Geometry: see drawing. Coordinates: mm, zero at the bounding-box minimum. A direction names the side the tool comes from. Coordinates: 2 decimals unless noted, no trailing zeros. Write each loop counter-clockwise with the first axis right and the second up, starting at its lowest first coordinate (ties: lowest second). Pieces come first, ordered by that corner, then holes. Notation, with made-up numbers: (58.25, 49.25) - (108.25, 49.25) arc R5 ccw to (108.25, 57.25) - close; hole circle Ø5 at (48.5, 77.5). An arc over 180 degrees is marked (long way). One line per question, with ' | ' between items. Start each with the question number.
Q1. Line query: line 1 (Z direction, x = 5.25, y = 0.85) (1 decimal); line 2 (X direction, y = 1.55, z = 7.25) (1 decimal); line 3 (X direction, y = 1, z = 3.25) (1 decimal). Output: solid intervals per line, ascending.
Q2. Cut plane A-A, the plane y = 0.55. Return loops of the section in (x, z) (1 decimal).
Q3. Draft query along X for the marked faces 1, 2, 3 and 4. Return one class per face: +X half, -X half, draft (parallel to the pull), parting line (faces both ways), or undercut.
Q4. Access query for the marked faces 5 and 6. Directions: +Z, -Z, +X, -X, +Y, -Y. A direction counts if a zero-diameter tool reaches every point of the face in a straight line with its end or side. Return the directions, or none.
Q5. Contact query for a flat-ended pin moving along its axis: P1, Ø1.3, axis at y = 1, z = 10, coming from the -X side. Output: stop coordinate, or through.
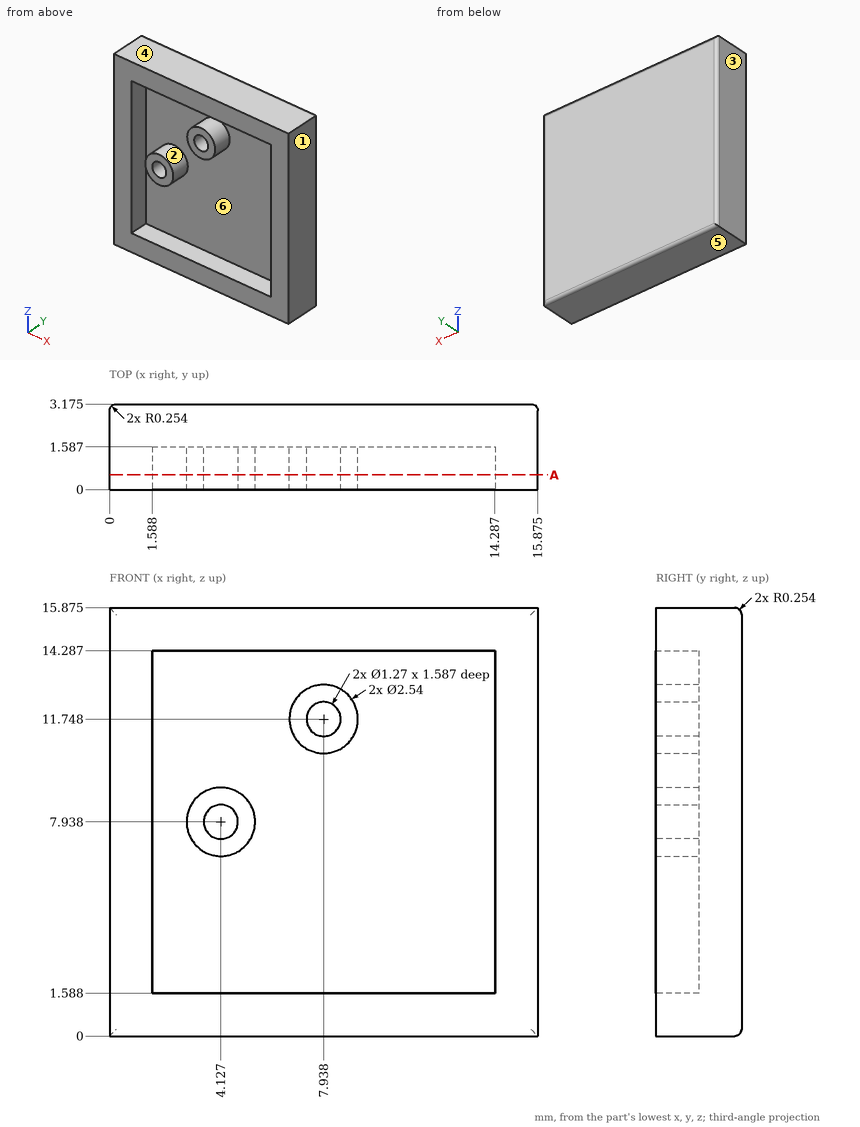
Reply:
1) line 1: z = 0 to 1.6, 7.3 to 8.5, 14.3 to 15.9 | line 2: x = 0 to 1.6, 3.1 to 5.2, 14.3 to 15.9 | line 3: x = 0 to 1.6, 14.3 to 15.9
2) outline: (0, 0) - (15.9, 0) - (15.9, 15.9) - (0, 15.9) - close; circle Ø2.5 at (4.1, 7.9); circle Ø2.5 at (7.9, 11.7); hole (1.6, 1.6) - (14.3, 1.6) - (14.3, 14.3) - (1.6, 14.3) - close; hole circle Ø1.3 at (4.1, 7.9); hole circle Ø1.3 at (7.9, 11.7)
3) face 1: +X half | face 2: undercut | face 3: -X half | face 4: draft
4) face 5: -Z, +X, -X, +Y, -Y | face 6: -Y
5) P1: stops at x = 0
